Design review of the part built by this model. Coordinates are the model's own, in mm. A direction names the side the tool comes from. Round coordinates to 2 decimals unless told otherwise and drop trailing zeros. Order: outer loops, then holes, each group sorted by start corner. A loop starts at its lowest first (then second) coordinate and runs counter-clockwise, first axis right, second up. Notation, with made-up numbers: (10.5, -2) - (24.5, -2) arc R30 cw to (24.5, 24) - close; hole circle Ø6 at (56, 36.5). An arc over 180 degrees is marked (long way). Write item = value, one per line.
from build123d import *

# Parameters (mm, degrees)
F0_W     = 101.6
F0_H     = 50.8
F1_DEPTH = 76.2
F2_R     = 6.35
F3_DEPTH = 76.201
F4_W     = 25.4
F4_H     = 25.4


with BuildPart() as f1:
    # F0 (on Front) → F1 (new body)
    with BuildSketch(Plane.XZ):
        Rectangle(F0_W, F0_H)
    extrude(amount=F1_DEPTH)

    # F2 (on face) → F3 (cut, through all)
    with BuildSketch(Plane.XZ.offset(76.2)):
        with Locations((-38.1, 12.7)):
            Circle(F2_R)
        with Locations((-38.1, -12.7)):
            Circle(F2_R)
        with Locations((38.1, -12.7)):
            Circle(F2_R)
        with Locations((38.1, 12.7)):
            Circle(F2_R)
    extrude(amount=-F3_DEPTH, mode=Mode.SUBTRACT)

    # F4 (on Top) → F5 (revolve)
    with BuildSketch(Plane.XY):
        with Locations((-12.7, -88.9)):
            Rectangle(F4_W, F4_H)
    revolve(axis=Axis((0, -54.245796, 0), (0, -1, 0)))


solid = f1.part
1) We need section C-C on y = -7. Write out the cut boundary in (x, z), and give its area (3 significant figures).
Findings:
outline = (-50.8, -25.4) - (50.8, -25.4) - (50.8, 25.4) - (-50.8, 25.4) - close; hole circle Ø12.7 at (-38.1, -12.7); hole circle Ø12.7 at (-38.1, 12.7); hole circle Ø12.7 at (38.1, -12.7); hole circle Ø12.7 at (38.1, 12.7)
area = 4,650 mm^2
2) We need section A-A on x = -38.1. Write out the cut boundary in (y, z), and give its area (3 significant figures).
Findings:
outline = (-76.2, -25.4) - (0, -25.4) - (0, -19.05) - (-76.2, -19.05) - close; (-76.2, -6.35) - (0, -6.35) - (0, 6.35) - (-76.2, 6.35) - close; (-76.2, 19.05) - (0, 19.05) - (0, 25.4) - (-76.2, 25.4) - close
area = 1,940 mm^2
3) For faces 1 (the flat face through (31, -76.2, 0)), 2 (the flat face through (-1, 0, 0)), list the 3-axis set-ups (+Z, -Z, +X, -X, +Y, -Y) from which the entire face can be reached by the end or side of a thin tool; tool diameter is ignored.
Findings:
face_1 = +X, -Y
face_2 = +Z, -Z, +X, -X, +Y
4) We need section D-D on z = 0. Write out the cut boundary in (x, y).
Findings:
outline = (-50.8, -76.2) - (-25.4, -76.2) - (-25.4, -101.6) - (25.4, -101.6) - (25.4, -76.2) - (50.8, -76.2) - (50.8, 0) - (-50.8, 0) - close
5) We need section B-B on z = -14. Write out the cut boundary in (x, y).
Findings:
outline = (-50.8, -76.2) - (-44.32, -76.2) - (-44.32, 0) - (-50.8, 0) - close; (-31.88, -76.2) - (-21.19, -76.2) - (-21.19, -101.6) - (21.19, -101.6) - (21.19, -76.2) - (31.88, -76.2) - (31.88, 0) - (-31.88, 0) - close; (44.32, -76.2) - (50.8, -76.2) - (50.8, 0) - (44.32, 0) - close
6) The part is to be moulded in two halves that separate along Z. For faces 3 (the cylindrical face through (-34.686, -38.633, 18.054)), 4 (the flat face through (0, -101.6, 0)), 5 (the flat face through (-1, -38, -25.4)), 6 (the cylindrical face through (5.506, -88.722, 24.796)), say which applies: released by +Z, released by -Z, zero draft, split by the parting line, or undercut.
Findings:
face_3 = undercut
face_4 = zero draft
face_5 = released by -Z
face_6 = split by the parting line
7) Clearance check with flat-ended pins moving along their axes: pin 1 Ø2 at (y, z) = (-77.5, -16.5) entering from -X; pin 2 Ø16.5 at (x, z) = (-38.1, 12.7) entering from -Y; pin 3 Ø7.5 at (x, z) = (38.1, 12.7) entering from -Y. State where each tip first meets the part, or that it passes through.
Findings:
pin_1 = -20.12
pin_2 = -76.2
pin_3 = through
8) To check wall thickness, follow L1, parallel to Z at x = -38.1, y = -29; L2, parallel to X at y = -64, z = 7.5; L3, parallel to X at y = -57, z = 12. State the ranges of each line that lie inside material, in increasing order. Write a range as from..to.
Findings:
L1 = -25.4..-19.05, -6.35..6.35, 19.05..25.4
L2 = -50.8..-41.74, -34.46..34.46, 41.74..50.8
L3 = -50.8..-44.41, -31.79..31.79, 44.41..50.8
